from build123d import *

# Parameters (mm, degrees)
SKETCH1_R           = 5
SKETCH1_R_2         = 3
BOSS_EXTRUDE1_DEPTH = 7
SKETCH2_R           = 3
BOSS_EXTRUDE2_DEPTH = 7
SKETCH3_W           = 16.288395929
SKETCH3_H           = 13.1
BOSS_EXTRUDE3_DEPTH = 4
SKETCH4_W           = 4.517614974
SKETCH4_H           = 7
CUT_EXTRUDE1_DEPTH  = 4
BOSS_EXTRUDE4_DEPTH = 4
BOSS_EXTRUDE5_DEPTH = 4
BOSS_EXTRUDE6_DEPTH = 19
BOSS_EXTRUDE7_DEPTH = 4
BOSS_EXTRUDE8_DEPTH = 8.1


with BuildPart() as part:
    # Sketch1 → Boss-Extrude1 (new body)
    with BuildSketch(Plane(origin=(0, 0, 0), x_dir=(1, 0, 0), z_dir=(0, 1, 0))):
        with Locations(Location((0, 0, 0), (0, 0, 270))):
            Circle(SKETCH1_R)
        with Locations(Location((0, 0, 0), (0, 0, 270))):
            Circle(SKETCH1_R_2, mode=Mode.SUBTRACT)
    extrude(amount=BOSS_EXTRUDE1_DEPTH)

    # Sketch2 → Boss-Extrude2 (add, through all)
    with BuildSketch(Plane(origin=(0, 7, 0), x_dir=(1, 0, 0), z_dir=(0, 1, 0))):
        with BuildLine():
            Line((4.582575695, -2), (34.582575695, -2))
            Line((34.582575695, -2), (34.582575695, 2))
            Line((34.582575695, 2), (4.582575695, 2))
            ThreePointArc((4.582575695, 2), (-5, 0), (4.582575695, -2))
        make_face()
        with Locations(Location((0, 0, 0), (0, 0, 270))):
            Circle(SKETCH2_R, mode=Mode.SUBTRACT)
    extrude(amount=-BOSS_EXTRUDE2_DEPTH)

    # Sketch3 → Boss-Extrude3 (add)
    with BuildSketch(Plane.XY.offset(2)):
        with Locations((21.920762757, 6.55)):
            Rectangle(SKETCH3_W, SKETCH3_H)
    extrude(amount=-BOSS_EXTRUDE3_DEPTH)

    # Sketch4 → Cut-Extrude1 (cut)
    with BuildSketch(Plane.XY.offset(2)):
        with Locations((32.323768208, 3.5)):
            Rectangle(SKETCH4_W, SKETCH4_H)
    extrude(amount=-CUT_EXTRUDE1_DEPTH, mode=Mode.SUBTRACT)

    # Sketch5 → Boss-Extrude4 (add)
    with BuildSketch(Plane.XY.offset(2)):
        Polygon((30.064960721, 13.1), (30.064960721, 0), (36.964960721, 0), (50.064960721, 13.1), (76.225581431, 13.1), (80.064960721, 19.75), (80.064960721, 26.4), (43.364960721, 26.4), align=None)
    extrude(amount=-BOSS_EXTRUDE4_DEPTH)

    # Sketch6 → Boss-Extrude5 (add)
    with BuildSketch(Plane.XY.offset(2)):
        Polygon((64.244452646, 36.204482672), (68.244452646, 36.204482672), (49.244452646, 3.295517328), (45.244452646, 3.295517328), align=None)
        Polygon((85.564960721, 36.204482672), (89.564960721, 36.204482672), (70.564960721, 3.295517328), (66.564960721, 3.295517328), align=None)
    extrude(amount=-BOSS_EXTRUDE5_DEPTH)

    # Sketch7 → Boss-Extrude6 (add)
    with BuildSketch(Plane.XY.offset(2)):
        Polygon((68.244452646, 36.204482672), (64.244452646, 36.204482672), (61.935051569, 32.204482672), (65.935051569, 32.204482672), align=None)
        Polygon((85.564960721, 36.204482672), (89.564960721, 36.204482672), (87.255559645, 32.204482672), (83.255559645, 32.204482672), align=None)
        Polygon((66.564960721, 3.295517328), (70.564960721, 3.295517328), (72.874361798, 7.295517328), (68.874361798, 7.295517328), align=None)
        Polygon((45.244452646, 3.295517328), (49.244452646, 3.295517328), (51.553853723, 7.295517328), (47.553853723, 7.295517328), align=None)
    extrude(amount=BOSS_EXTRUDE6_DEPTH)

    # Sketch8 → Boss-Extrude7 (add)
    with BuildSketch(Plane.XY.offset(21)):
        Polygon((64.244452646, 36.204482672), (68.244452646, 36.204482672), (49.244452646, 3.295517328), (45.244452646, 3.295517328), align=None)
        Polygon((85.564960721, 36.204482672), (89.564960721, 36.204482672), (70.564960721, 3.295517328), (66.564960721, 3.295517328), align=None)
    extrude(amount=-BOSS_EXTRUDE7_DEPTH)

    # Sketch9 → Boss-Extrude8 (add)
    with BuildSketch(Plane(origin=(0, 0, -2), x_dir=(-1, 0, 0), z_dir=(0, 0, -1))):
        Polygon((-54.905073356, 13.1), (-62.583831936, 26.4), (-83.95273694, 26.483825938), (-76.273978359, 13.183825938), align=None)
    extrude(amount=BOSS_EXTRUDE8_DEPTH)


solid = part.part
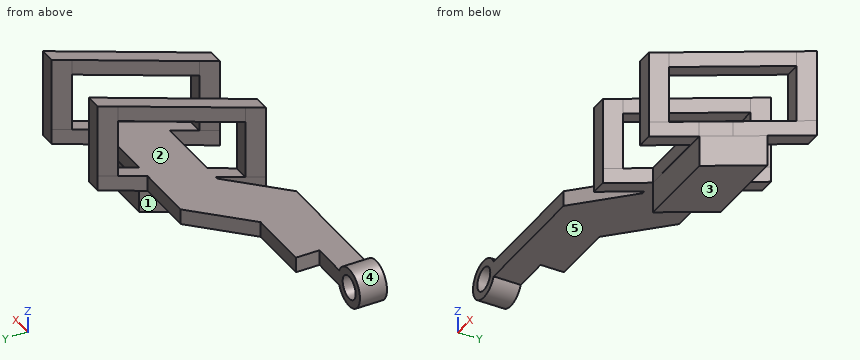
Part model, mm, in its own coordinate system. Face numbers are marked on the shaded views. A direction names the side the tool comes from. Coordinates: 2 decimals unless noted, no trailing zeros. Order: outer loops, then holes, each group sorted by start corner. A loop starts at its lowest first (then second) coordinate and runs counter-clockwise, first axis right, second up. Notation, with made-up numbers: M -20.5,-36.75 L -2.5,-36.75 A22 cw -2.5,-25.75 Z; hole C -34,10 d11. An arc over 180 degrees is marked long. One line per question, with ' | ' between items.
Q1. 3-axis set-ups, long thin cutter, end or side, ignore diameter. For the marked faces 4 and 5: which of +Z, -Z, +X, -X, +Y, -Y reach the whole face in a straight line?
A:
face 4: +Y, -Y | face 5: -Z, +Y
Q2. Slice it at A-A (x = 0). Give the cut face in (y, z).
A:
outline: M 0,-5 L 7,-5 L 7,-3 L 0,-3 Z; M 0,3 L 7,3 L 7,5 L 0,5 Z
Q3. Drill centre lines: line 1 (X direction, y = 4.75, z = 0); line 2 (X direction, y = 12, z = 0.5); line 3 (Z direction, x = 65, y = 34.5). Where is each one in solid material? Low to high.
A:
line 1: x = -5 to -3, 3 to 41.71, 46.08 to 50.08, 67.4 to 71.4 | line 2: x = 13.78 to 48.96, 50.27 to 54.27, 71.59 to 75.59 | line 3: z = -2 to 21
Q4. Slice it at D-D (y = 11). Give the cut face in (x, z).
A:
outline: M 13.78,-2 L 47.96,-2 L 47.96,2 L 13.78,2 Z; M 49.69,-2 L 53.69,-2 L 53.69,2 L 49.69,2 Z; M 49.69,17 L 53.69,17 L 53.69,21 L 49.69,21 Z; M 71.01,-2 L 75.01,-2 L 75.01,2 L 71.01,2 Z; M 71.01,17 L 75.01,17 L 75.01,21 L 71.01,21 Z
Q5. Pin check, flat tips, straight feed: P1, Ø11, axis at x = 63.5, y = 7.5, coming from the -Z side; P2, Ø2, axis at x = 24.5, z = -0.5, coming from the +Y side; P3, Ø3, axis at x = 59.5, z = 0, coming from the -Y side; P4, Ø3, axis at x = 75, y = 29.5, coming from the +Z side. Stop position of each tip, or through.
A:
P1: stops at z = -2 | P2: stops at y = 13.1 | P3: stops at y = 13.1 | P4: passes through
Q6. Slice it at C-C (z = 0). Give the cut face in (x, y), and give its area (3 significant figures).
A:
outline: M -5,0 L -3,0 L -3,7 L -5,7 Z; M 3,0 L 36.96,0 L 50.06,13.1 L 50.91,13.1 L 45.24,3.3 L 49.24,3.3 L 54.91,13.1 L 72.23,13.1 L 66.56,3.3 L 70.56,3.3 L 89.56,36.2 L 85.56,36.2 L 79.9,26.4 L 62.58,26.4 L 68.24,36.2 L 64.24,36.2 L 58.58,26.4 L 43.36,26.4 L 30.06,13.1 L 13.78,13.1 L 13.78,7 L 3,7 Z | area: 1,210 mm^2
Q7. Two-plate mould, pull along Z, no slides. Class the marked faces 1, 2 and 3: +Z half, -Z half, draft (parallel to the pull), parting line (faces both ways), or undercut.
A:
face 1: draft | face 2: undercut | face 3: -Z half
Q8. Slice it at B-B (z = 7). Give the cut face in (x, y).
A:
outline: M 45.24,3.3 L 49.24,3.3 L 51.55,7.3 L 47.55,7.3 Z; M 61.94,32.2 L 65.94,32.2 L 68.24,36.2 L 64.24,36.2 Z; M 66.56,3.3 L 70.56,3.3 L 72.87,7.3 L 68.87,7.3 Z; M 83.26,32.2 L 87.26,32.2 L 89.56,36.2 L 85.56,36.2 Z
